Here's how the part is built. I have some questions about the finished solid (model axes, mm). Face numbers are marked on the shaded views. A direction names the side the tool comes from. Round coordinates to 2 decimals unless told otherwise and drop trailing zeros. Order: outer loops, then holes, each group sorted by start corner. A loop starts at its lowest first (then second) coordinate and runs counter-clockwise, first axis right, second up. Notation, with made-up numbers: (46.5, 10) - (99.5, 10) arc R14 cw to (99.5, 32) - close; hole circle Ø5 at (89.5, -16.75). An arc over 180 degrees is marked (long way). One line per item, written item: value.
from build123d import *

# Parameters (mm, degrees)
F0_R      = 15
F1_DEPTH  = 12
F4_R      = 3
F5_DEPTH  = 3
F6_R      = 4.5
F7_DEPTH  = 1.5
F9_DEPTH  = 4
F10_R     = 1.5
F11_DEPTH = 18
F12_R     = 7.5
F13_DEPTH = 10.4
F14_R     = 12.5
F15_DEPTH = 2.4
F16_R     = 5.5
F16_R_2   = 1
F17_DEPTH = 2.4


with BuildPart() as f1:
    # F0 (on Top) → F1 (new body)
    with BuildSketch(Plane.XY):
        Circle(F0_R)
    extrude(amount=F1_DEPTH)

    # F2 (on Front) → F3 (revolve)
    with BuildSketch(Plane.XZ):
        Polygon((11, 14.4), (0, 14.4), (0, 12), (15, 12), (15, 13), align=None)
    revolve(axis=Axis((0, 0, 13.2), (0, 0, -1)))

    # F4 (on face) → F5 (cut)
    with BuildSketch(Plane.XY.offset(14.4)):
        with Locations((0, 9)):
            Circle(F4_R)
        with Locations((-7.794229, 4.5)):
            Circle(F4_R)
        with Locations((-7.794229, -4.5)):
            Circle(F4_R)
        with Locations((0, -9)):
            Circle(F4_R)
        with Locations((7.794229, -4.5)):
            Circle(F4_R)
        with Locations((7.794229, 4.5)):
            Circle(F4_R)
    extrude(amount=-F5_DEPTH, mode=Mode.SUBTRACT)

    # F6 (on face) → F7 (join)
    with BuildSketch(Plane.XY.offset(14.4)):
        Circle(F6_R)
    extrude(amount=F7_DEPTH)

    # F8 (on face) → F9 (join)
    with BuildSketch(Plane.XY.offset(15.9)):
        with BuildLine():
            Line((3.35, -3.00458), (3.35, 3.00458))
            ThreePointArc((3.35, 3.00458), (0, 4.5), (-3.35, 3.00458))
            Line((-3.35, 3.00458), (-3.35, -3.00458))
            ThreePointArc((-3.35, -3.00458), (0, -4.5), (3.35, -3.00458))
        make_face()
    extrude(amount=F9_DEPTH)

    # F10 (on face) → F11 (join)
    with BuildSketch(Plane.XY.offset(19.9)):
        Circle(F10_R)
    extrude(amount=F11_DEPTH)

    # F12 (on face) → F13 (join)
    with BuildSketch(Plane(origin=(0, 0, 0), x_dir=(1, 0, 0), z_dir=(0, 0, -1))):
        Circle(F12_R)
    extrude(amount=F13_DEPTH)

    # F14 (on face) → F15 (join)
    with BuildSketch(Plane(origin=(0, 0, -10.4), x_dir=(1, 0, 0), z_dir=(0, 0, -1))):
        Circle(F14_R)
    extrude(amount=F15_DEPTH)

    # F16 (on face) → F17 (cut)
    with BuildSketch(Plane(origin=(0, 0, -12.8), x_dir=(1, 0, 0), z_dir=(0, 0, -1))):
        Circle(F16_R)
        with Locations((10, 0)):
            Circle(F16_R_2)
        with Locations((-5, 8.660254)):
            Circle(F16_R_2)
        with Locations((-5, -8.660254)):
            Circle(F16_R_2)
    extrude(amount=-F17_DEPTH, mode=Mode.SUBTRACT)


solid = f1.part
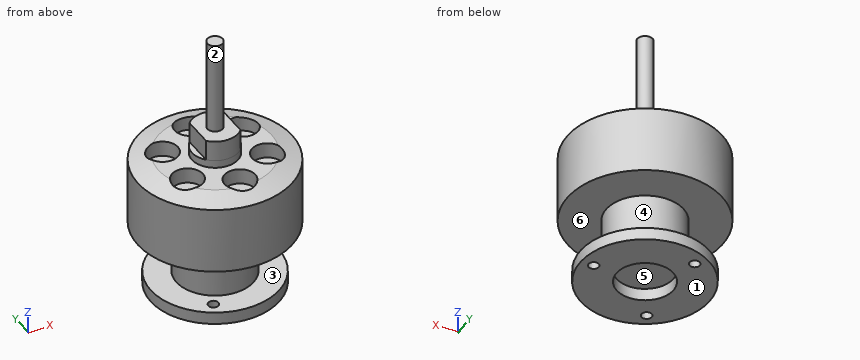
Q1. Which directions (+Z, -Z, +X, -X, +Y, -Y) give clear straight access to the entire face, cutting with the end or side of a thin tool? Please do the marked faces 1, 2 and 3.
Results list:
face 1: -Z, +X, -X, +Y, -Y
face 2: +Z
face 3: none
Q2. We'd pull the mould along Y, two halves only. Please class the marked faces 4, 5 and 6: released by +Y, released by -Y, zero draft, split by the parting line, or undercut.
Results list:
face 4: split by the parting line
face 5: undercut
face 6: zero draft
Q3. If I drill on line 1 along X through (y, z) = (0, -11.8); line 2 along Y through (x, z) = (0, 12.15); line 3 along Z through (x, y) = (-2.5, 10.5), over which ranges is the centre line in solid material (lowest first)?
Results list:
line 1: -12.5 to -5.5, 5.5 to 9, 11 to 12.5
line 2: -15 to -12, -6 to 6, 12 to 15
line 3: -12.8 to -10.4, 0 to 11.4
Q4. If we section it at C-C, the plane z = 4: Please give me the cut outline in (x, y), then the cut area to 3 significant figures.
Results list:
outline: circle Ø30 at (0, 0)
area: 707 mm²
Q5. Will these pins go through, and if not, where does the flat tip stop? pin 1 (3 mm diameter, centred on y = -1, z = 17.5, fed in from +X); pin 2 (6.5 mm diameter, centred on x = -1.5, y = -8.5, fed in from +Z); pin 3 (0.6 mm diameter, centred on x = 4, y = 0.5, fed in from +Z); pin 4 (10 mm diameter, centred on y = -9.5, z = 31.5, fed in from -X).
Results list:
pin 1: x = 3.35
pin 2: z = 14.4
pin 3: z = 15.9
pin 4: through
Q6. If we section it at D-D, the plane z = -2: Please give me the cut outline in (x, y), then the cut area to 3 significant figures.
Results list:
outline: circle Ø15 at (0, 0)
area: 177 mm²
